from build123d import *

# Parameters (mm, degrees)
PAD_DEPTH    = 15
SKETCH001_R  = 1.65
POCKET_DEPTH = 6.001


with BuildPart() as part:
    # Sketch → Pad (new body)
    with BuildSketch(Plane.XY):
        with BuildLine():
            ThreePointArc((2.55, 0), (0, 2.55), (-2.55, 0))
            Line((-2.55, 0), (-8.5, 0))
            Line((-8.5, 0), (-8.5, 6))
            Line((-8.5, 6), (8.5, 6))
            Line((8.5, 6), (8.5, 0))
            Line((2.55, 0), (8.5, 0))
        make_face()
    extrude(amount=PAD_DEPTH)

    # Sketch001 → Pocket (cut, through all)
    with BuildSketch(Plane.XZ):
        with Locations((-5.5, 3)):
            Circle(SKETCH001_R)
        with Locations((-5.5, 12)):
            Circle(SKETCH001_R)
        with Locations((5.5, 12)):
            Circle(SKETCH001_R)
        with Locations((5.5, 3)):
            Circle(SKETCH001_R)
    extrude(amount=-POCKET_DEPTH, mode=Mode.SUBTRACT)


solid = part.part
CAD build for the part. Positions are in the model's coordinates, mm. Give positions to 0.01 mm unless a question says otherwise; leave off trailing zeros. Loops run counter-clockwise (first coordinate to the right, second up) from the corner with the lowest first, then second, coordinate; pieces in that order, holes last. Notation, with made-up numbers: M -7,67 L -3,67 A22 cw -3,74 Z; hole C 37,81 d2. An arc over 180 degrees is marked long. One line per question, with ' | ' between items. Start each with the question number.
1. Saw through at B-B on z = 12. Give the cut face in (x, y).
2. Flat gauge pins, fed straight in: pin 1 (1 mm diameter, centred on x = -6, z = 11.5, fed in from +Y) (3 decimals); pin 2 (1.5 mm diameter, centred on x = 0.5, z = 12.5, fed in from -Y); pin 3 (1.5 mm diameter, centred on x = -1, z = 5.5, fed in from -Y). Where does each tip first touch, or does it go through?
3. Saw through at D-D on y = 3.7. Give the cut face in (x, z).
4. Saw through at C-C on y = 0.8. Give the cut face in (x, z), plus the area to 3 significant figures.
5. Probe L1, parallel to Z at x = 5.5, y = 3.1; L2, parallel to X at y = 1.3, z = 13; L3, parallel to X at y = 1.1, z = 11.75. List the from-to ranges inside material, lowest first. Write a range as from..to.
6. Two-plate mould, pull along X, no slides. Class faces 1 (the face through (0, 3, 15)), 2 (the face through (4.19, 2.96, 11)), 3 (the face through (-6.716, 2.958, 4.115)), 4 (the face through (8.5, 3, 7)): pulls with the +X half, pulls with the -X half, needs draft (parallel to the pull), parting line crosses it, or undercut.
7. Saw through at A-A on x = -5.5. Give the cut face in (y, z).
Result sheet:
1) outline: M -8.5,0 L -7.15,0 L -7.15,6 L -8.5,6 Z; M -3.85,0 L -2.55,0 A2.55 cw 2.55,0 L 3.85,0 L 3.85,6 L -3.85,6 Z; M 7.15,0 L 8.5,0 L 8.5,6 L 7.15,6 Z
2) pin 1: passes through | pin 2: stops at y = 2.22 | pin 3: stops at y = 1.85
3) outline: M -8.5,0 L 8.5,0 L 8.5,15 L -8.5,15 Z; hole C -5.5,3 d3.3; hole C -5.5,12 d3.3; hole C 5.5,3 d3.3; hole C 5.5,12 d3.3
4) outline: M -8.5,0 L -2.42,0 L -2.42,15 L -8.5,15 Z; M 2.42,0 L 8.5,0 L 8.5,15 L 2.42,15 Z; hole C -5.5,3 d3.3; hole C -5.5,12 d3.3; hole C 5.5,3 d3.3; hole C 5.5,12 d3.3 | area: 148 mm^2
5) L1: z = 0..1.35, 4.65..10.35, 13.65..15 | L2: x = -8.5..-6.81, -4.19..-2.19, 2.19..4.19, 6.81..8.5 | L3: x = -8.5..-7.13, -3.87..-2.3, 2.3..3.87, 7.13..8.5
6) face 1: needs draft | face 2: undercut | face 3: undercut | face 4: pulls with the +X half
7) outline: M 0,0 L 6,0 L 6,1.35 L 0,1.35 Z; M 0,4.65 L 6,4.65 L 6,10.35 L 0,10.35 Z; M 0,13.65 L 6,13.65 L 6,15 L 0,15 Z
